Source: CAD feature listing. Evaluate the final solid. Frame: model axes, mm. Face numbers are marked on the shaded views. Round coordinates to 2 decimals unless told otherwise and drop trailing zeros. Write each loop counter-clockwise with the first axis right and the second up, starting at its lowest first coordinate (ties: lowest second). Pieces come first, ordered by that corner, then holes. Notation, with made-up numbers: M 59,73.25 L 93,73.25 A17 ccw 93,78.25 Z; hole C 1.25,-27.5 d3. An arc over 180 degrees is marked long. Use a Markdown table: item, result.
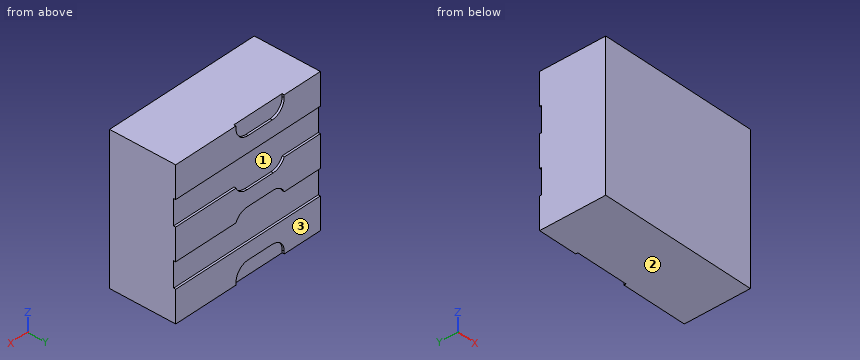
```python
from build123d import *

# Parameters (mm, degrees)
SKETCH1_W           = 6
SKETCH1_H           = 2.5
BOSS_EXTRUDE1_DEPTH = 2.75
SKETCH3_OUTSIDE_W   = 9.702
SKETCH3_OUTSIDE_H   = 9.202
SKETCH3_OUTSIDE_W_2 = 4
SKETCH3_OUTSIDE_H_2 = 0.6
CUT_EXTRUDE1_DEPTH  = 0.08
SKETCH7_W           = 1.5
SKETCH7_H           = 1.2
SKETCH7_W_2         = 2.5
BOSS_EXTRUDE3_DEPTH = 0.2
FILLET2_R           = 0.5


with BuildPart() as part:
    # Sketch1 → Boss-Extrude1 (new, symmetric)
    with BuildSketch(Plane.XY):
        Rectangle(SKETCH1_W, SKETCH1_H)
    extrude(amount=BOSS_EXTRUDE1_DEPTH, both=True)

    # Sketch3 outside → Cut-Extrude1 (cut)
    with BuildSketch(Plane(origin=(0, 1.25, 0), x_dir=(1, 0, 0), z_dir=(0, 1, 0))):
        Rectangle(SKETCH3_OUTSIDE_W, SKETCH3_OUTSIDE_H)
        with Locations((0, 1.85)):
            Rectangle(SKETCH3_OUTSIDE_W_2, SKETCH3_OUTSIDE_H_2, mode=Mode.SUBTRACT)
        with Locations((0, -1.85)):
            Rectangle(SKETCH3_OUTSIDE_W_2, SKETCH3_OUTSIDE_H_2, mode=Mode.SUBTRACT)
        Rectangle(SKETCH3_OUTSIDE_W_2, SKETCH3_OUTSIDE_H_2, mode=Mode.SUBTRACT)
    extrude(amount=-CUT_EXTRUDE1_DEPTH, mode=Mode.SUBTRACT)

    # Sketch7 → Boss-Extrude3 (add)
    with BuildSketch(Plane(origin=(0, 1.25, 0), x_dir=(1, 0, 0), z_dir=(0, 1, 0))):
        with Locations((-2.25, 2.15)):
            Rectangle(SKETCH7_W, SKETCH7_H)
        with Locations((-2.25, -2.15)):
            Rectangle(SKETCH7_W, SKETCH7_H)
        with Locations((1.75, 2.15)):
            Rectangle(SKETCH7_W_2, SKETCH7_H)
        with Locations((1.75, -2.15)):
            Rectangle(SKETCH7_W_2, SKETCH7_H)
        with Locations((-2.25, 0)):
            Rectangle(SKETCH7_W, SKETCH7_H)
        with Locations((1.75, 0)):
            Rectangle(SKETCH7_W_2, SKETCH7_H)
    extrude(amount=-BOSS_EXTRUDE3_DEPTH)

    # Fillet2
    # the kernel refuses this fillet: 0.5 mm, written as the material it adds along each edge
    with BuildSketch(Plane(origin=(0.5, 1.25, -2.15), x_dir=(-1, 0, 0), z_dir=(0, -1, 0)), Plane(origin=(0.5, -0.08, 2.15), x_dir=(-1, 0, 0), z_dir=(0, 1, 0)), Plane(origin=(-1.5, 1.25, -2.15), x_dir=(0, 0, -1), z_dir=(0, -1, 0)), Plane(origin=(-1.5, -0.08, 2.15), x_dir=(0, 0, 1), z_dir=(0, 1, 0))) as fillet2_piece_1:
        with BuildLine():
            CenterArc((FILLET2_R, FILLET2_R), FILLET2_R, 180, 90)
            Line((0, FILLET2_R), (-FILLET2_R * 0.02, FILLET2_R))
            Line((-FILLET2_R * 0.02, FILLET2_R), (-FILLET2_R * 0.02, -FILLET2_R * 0.02))
            Line((-FILLET2_R * 0.02, -FILLET2_R * 0.02), (FILLET2_R, -FILLET2_R * 0.02))
            Line((FILLET2_R, -FILLET2_R * 0.02), (FILLET2_R, 0))
        make_face()
    extrude(amount=1.33)
    with BuildSketch(Plane(origin=(-1.5, 0.024356076, -0.3), x_dir=(1, 0, 0), z_dir=(0, 1, 0)), Plane(origin=(0.5, 0.024356076, 0.3), x_dir=(-1, 0, 0), z_dir=(0, 1, 0))) as fillet2_piece_2:
        with BuildLine():
            CenterArc((0.458257569, 0.5), FILLET2_R, 203.578178478, 66.421821522)
            Line((0, 0.3), (-0.009165151, 0.296))
            ThreePointArc((-0.009165151, 0.296), (-0.01, 0.15), (-0.01, 0))
            Line((-0.01, 0), (0, -0.01))
            Line((0, -0.01), (0.458257569, -0.01))
            Line((0.458257569, -0.01), (0.458257569, 0))
        make_face()
    extrude(amount=1.225643924)
    with BuildSketch(Plane(origin=(-1.5, 1.25, 0.3), x_dir=(0, 0, 1), z_dir=(0, -1, 0)), Plane(origin=(0.5, 1.25, -0.3), x_dir=(0, 0, -1), z_dir=(0, -1, 0))) as fillet2_piece_3:
        with BuildLine():
            CenterArc((0.5, -0.458257569), FILLET2_R, 113.578178478, 66.421821522)
            Line((0, -0.458257569), (-0.01, -0.458257569))
            Line((-0.01, -0.458257569), (-0.01, 0))
            Line((-0.01, 0), (0, 0.01))
            ThreePointArc((0, 0.01), (0.15, 0.01), (0.296, 0.009165151))
            Line((0.296, 0.009165151), (0.3, 0))
        make_face()
    extrude(amount=1.225643924)


solid = part.part
```
Q1. Section B-B on z = -0.7. Return loops of the section in (x, y).
Results are:
| item | result |
|---|---|
| outline | M -3,-1.25 L 3,-1.25 L 3,1.17 L -3,1.17 Z |
Q2. Mould query, pull axis Z, two halves, no side actions, for the marked faces 1, 2 and 3. Classes: +Z half, -Z half, draft (parallel to the pull), parting line (faces both ways), or undercut.
Results are:
| item | result |
|---|---|
| face 1 | undercut |
| face 2 | -Z half |
| face 3 | draft |
Q3. Section A-A on x = -0.45. Return loops of the section in (y, z), plus the area to 3 significant figures.
Results are:
| item | result |
|---|---|
| outline | M -1.25,-2.75 L 1.17,-2.75 L 1.17,-2.15 L 1.25,-2.15 L 1.25,-1.55 L 1.17,-1.55 L 1.17,-0.3 L 1.25,-0.3 L 1.25,0.3 L 1.17,0.3 L 1.17,1.55 L 1.25,1.55 L 1.25,2.15 L 1.17,2.15 L 1.17,2.75 L -1.25,2.75 Z |
| area | 13.5 mm^2 |
Q4. First-contact query: pin 1 Ø0.5 at (x, z) = (0, -2.5) entering from +Y. Flat tip, straight axial feed; report the tip coordinate or a pass-through.
Results are:
| item | result |
|---|---|
| pin 1 | y = 1.17 |
Q5. Line query: L1, parallel to Y at x = 1.85, z = -0.9. Output: solid intervals per line, ascending.
Results are:
| item | result |
|---|---|
| L1 | -1.25 to 1.17 |
Q6. Section C-C on x = -1.2. Return loops of the section in (y, z), plus the area to 3 significant figures.
Results are:
| item | result |
|---|---|
| outline | M -1.25,-2.75 L 1.17,-2.75 L 1.17,-2.19 L 1.25,-2.19 L 1.25,-1.55 L 1.17,-1.55 L 1.17,-0.33 L 1.25,-0.33 L 1.25,0.33 L 1.17,0.33 L 1.17,1.55 L 1.25,1.55 L 1.25,2.19 L 1.17,2.19 L 1.17,2.75 L -1.25,2.75 Z |
| area | 13.5 mm^2 |
